For this review, use the dimensioned drawing (mm, ordinates from the lowest corner) and the shaded views. A direction names the side the tool comes from. Round coordinates to 2 decimals unless told otherwise and drop trailing zeros. Write each loop counter-clockwise with the first axis right and the second up, starting at its lowest first coordinate (ties: lowest second). Pieces come first, ordered by that corner, then holes. Notation, with made-up numbers: (35, 26.25) - (75, 26.25) arc R16 ccw to (75, 52.25) - close; hole circle Ø8 at (7, 66). An arc over 180 degrees is marked (long way). Write each question's results on one line, items separated by ' | '.
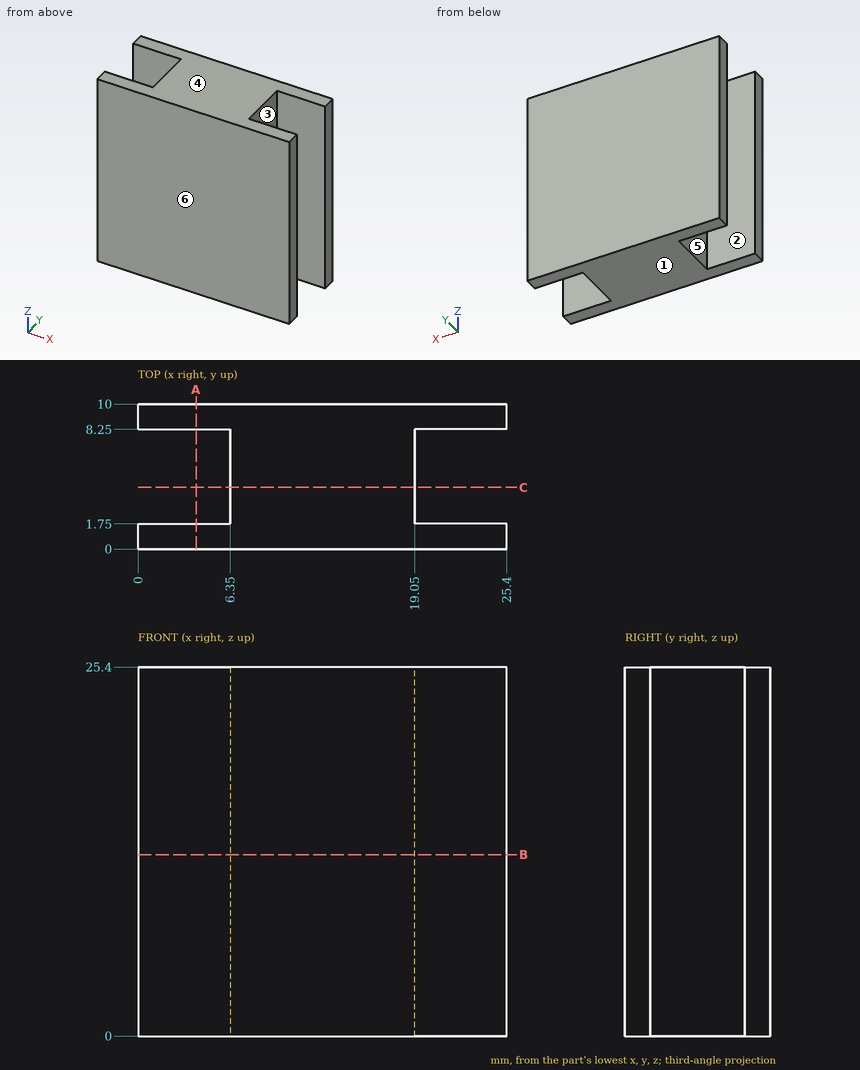
Q1. Insertion check: P1, Ø5, axis at y = 6, z = 14.5, coming from the +X side; P2, Ø1, axis at y = 6.5, z = 14.5, coming from the +X side; P3, Ø2, axis at y = 4, z = 14.5, coming from the -X side. Each pin has a flat end and moves straight along its axis. Give the tip position at first contact, or say it passes through.
Evaluation:
P1: stops at x = 25.4 | P2: stops at x = 19.05 | P3: stops at x = 6.35
Q2. For probe 1 along Y at (x, z) = (4.5, 4.25); probe 2 along X at (y, z) = (2.5, 4.25), list the stretches that pass through material, from the lowest coordinate up.
Evaluation:
probe 1: y = 0 to 1.75, 8.25 to 10 | probe 2: x = 6.35 to 19.05
Q3. We need section A-A (x = 4). State the section outline as (y, z) points, plus the area to 3 significant figures.
Evaluation:
outline: (0, 0) - (1.75, 0) - (1.75, 25.4) - (0, 25.4) - close; (8.25, 0) - (10, 0) - (10, 25.4) - (8.25, 25.4) - close | area: 88.9 mm^2
Q4. We need section B-B (z = 12.5). State the section outline as (x, y) points, plus the area to 3 significant figures.
Evaluation:
outline: (0, 0) - (25.4, 0) - (25.4, 1.75) - (19.05, 1.75) - (19.05, 8.25) - (25.4, 8.25) - (25.4, 10) - (0, 10) - (0, 8.25) - (6.35, 8.25) - (6.35, 1.75) - (0, 1.75) - close | area: 171 mm^2
Q5. The part is to be moulded in two halves that separate along Y. For the marked faces 4, 5 and 6, say which applies: released by +Y, released by -Y, zero draft, split by the parting line, or undercut.
Evaluation:
face 4: zero draft | face 5: undercut | face 6: released by -Y
Q6. We need section C-C (y = 4.25). State the section outline as (x, z) points, plus the area to 3 significant figures.
Evaluation:
outline: (6.35, 0) - (19.05, 0) - (19.05, 25.4) - (6.35, 25.4) - close | area: 323 mm^2
Q7. Tool access review of the marked faces 1, 2 and 3: name each direction out of +Z, -Z, +X, -X, +Y, -Y from which nothing blocks a thin tool from reaching the whole face with its end or side.
Evaluation:
face 1: -Z, +X, -X, +Y, -Y | face 2: +Z, -Z, -X | face 3: +Z, -Z, +X
